```python
from build123d import *

# Parameters (mm, degrees)
BOSS_EXTRUDE1_DEPTH = 3
BOSS_EXTRUDE2_DEPTH = 15
BOSS_EXTRUDE3_DEPTH = 3
SKETCH5_R           = 2.25
CUT_EXTRUDE1_DEPTH  = 3
SKETCH6_R           = 2.6
CUT_EXTRUDE2_DEPTH  = 3
FILLET1_R           = 1


with BuildPart() as part:
    # Sketch2 → Boss-Extrude1 (new body)
    with BuildSketch(Plane(origin=(0, 0, 0), x_dir=(0, 0, -1), z_dir=(1, 0, 0))):
        Polygon((0, 0), (0, 40), (-5, 40), (-19, 5), (-19, 0), align=None)
    extrude(amount=BOSS_EXTRUDE1_DEPTH)

    # Sketch3 → Boss-Extrude2 (add)
    with BuildSketch(Plane(origin=(3, 0, 0), x_dir=(0, 0, -1), z_dir=(1, 0, 0))):
        Polygon((-19, 0), (-19, 3), (-3, 3), (-3, 40), (0, 40), (0, 0), align=None)
    extrude(amount=BOSS_EXTRUDE2_DEPTH)

    # Sketch4 → Boss-Extrude3 (add)
    with BuildSketch(Plane(origin=(18, 0, 0), x_dir=(0, 0, -1), z_dir=(1, 0, 0))):
        Polygon((-19, 0), (0, 0), (0, 40), (-5, 40), (-19, 5), align=None)
    extrude(amount=BOSS_EXTRUDE3_DEPTH)

    # Sketch5 → Cut-Extrude1 (cut)
    with BuildSketch(Plane(origin=(0, 0, 0), x_dir=(-1, 0, 0), z_dir=(0, 0, -1))):
        with Locations((-10.5, 30.5)):
            Circle(SKETCH5_R)
    extrude(amount=-CUT_EXTRUDE1_DEPTH, mode=Mode.SUBTRACT)

    # Sketch6 → Cut-Extrude2 (cut)
    with BuildSketch(Plane.XZ):
        with Locations(Location((10.5, 10, 0), (0, 0, 270))):
            Circle(SKETCH6_R)
    extrude(amount=-CUT_EXTRUDE2_DEPTH, mode=Mode.SUBTRACT)

    # Fillet1
    fillet1_edges = [part.edges().sort_by_distance(p)[0] for p in [
        (3, 22.5, 12),
        (3, 4, 19),
        (3, 40, 4),
        (3, 21.5, 3),
        (10.5, 40, 3),
        (3, 3, 11),
        (10.5, 3, 19),
        (18, 21.5, 3),
        (18, 3, 11),
        (18, 40, 4),
        (18, 22.5, 12),
        (18, 4, 19),
        (21, 20, 0),
        (21, 40, 2.5),
        (21, 22.5, 12),
        (21, 2.5, 19),
        (21, 0, 9.5),
        (0, 2.5, 19),
        (12.75, 30.5, 0),
        (0, 22.5, 12),
        (10.5, 0, 12.6),
        (0, 40, 2.5),
        (0, 20, 0),
        (0, 0, 9.5),
        (10.5, 0, 19),
        (10.5, 40, 0),
        (10.5, 0, 0),
    ]]
    fillet(fillet1_edges, radius=FILLET1_R)


solid = part.part
```
Source: CAD feature listing. Evaluate the final solid. Frame: model axes, mm. A direction names the side the tool comes from. Give positions to 0.01 mm unless a question says otherwise; leave off trailing zeros. Loops run counter-clockwise (first coordinate to the right, second up) from the corner with the lowest first, then second, coordinate; pieces in that order, holes last. Notation, with made-up numbers: (60, 29.25) -> (109, 29.25) arc R16 cw to (109, 33.25) -> close; hole circle Ø11 at (74, 57). An arc over 180 degrees is marked (long way). Use a Markdown table: item, result. Add a question column.
(1) Ray query, line 1 (X direction, y = 23, z = 6.75); line 2 (X direction, y = 2.45, z = 10); line 3 (Y direction, x = 5.5, z = 6.75). Return the intervals inside material, ascending.
(2) First-contact query: pin 1 Ø4 at (x, z) = (8.5, 13) entering from +Y; pin 2 Ø8 at (x, y) = (9.5, 33) entering from +Z; pin 3 Ø6 at (x, z) = (18.5, 9) entering from -Y; pin 4 Ø6 at (x, z) = (10.5, 10) entering from -Y. Flat tips, straight axial feed; report the tip coordinate or a pass-through.
(3) Section query B-B (x = 5). Output: boundary loops of the cut face in (y, z), then the cut area to 3 significant figures.
(4) Section query A-A (x = 10.5). Output: boundary loops of the cut face in (y, z), then the cut area to 3 significant figures.
(5) Access query for faces 1 (the face through (0.301, 2.972, 18.715)), 2 (the face through (2.699, 4.493, 18.715)). Directions: +Z, -Z, +X, -X, +Y, -Y. A direction counts if a zero-diameter tool reaches every point of the face in a straight line with its end or side. Return the directions, or none.
(6) Pull-direction query (X, two-part tool) for faces 3 (the face through (1.493, 22.745, 11.902)), 4 (the face through (21, 16, 8)), 5 (the face through (2.7, 22.15, 11.83)), 6 (the face through (8.193, 1.986, 8.8)); classes: +X half, -X half, draft (parallel to the pull), parting line (faces both ways), or undercut.
Checked values:
| question | item | result |
|---|---|---|
| 1 | line 1 | 0 to 3, 18 to 21 |
| 1 | line 2 | 0 to 7.9, 13.1 to 21 |
| 1 | line 3 | 0 to 3 |
| 2 | pin 1 | y = 3 |
| 2 | pin 2 | z = 3 |
| 2 | pin 3 | y = 0 |
| 2 | pin 4 | y = 0.2 |
| 3 | outline | (0, 1) arc R1 ccw to (1, 0) -> (39, 0) arc R1 ccw to (40, 1) -> (40, 2) arc R1 ccw to (39, 3) -> (3, 3) -> (3, 18) arc R1 ccw to (2, 19) -> (1, 19) arc R1 ccw to (0, 18) -> close |
| 3 | area | 167 mm^2 |
| 4 | outline | (0, 1) arc R1 ccw to (1, 0) -> (27.25, 0) arc R1 ccw to (28.25, 1) -> (28.25, 3) -> (3, 3) -> (3, 7.4) -> (1, 7.4) arc R1 ccw to (0, 6.4) -> close; (0, 13.6) arc R1 ccw to (1, 12.6) -> (3, 12.6) -> (3, 18) arc R1 ccw to (2, 19) -> (1, 19) arc R1 ccw to (0, 18) -> close; (32.75, 1) arc R1 ccw to (33.75, 0) -> (39, 0) arc R1 ccw to (40, 1) -> (40, 2) arc R1 ccw to (39, 3) -> (32.75, 3) -> close |
| 4 | area | 137 mm^2 |
| 5 | face 1 | +Z, -X, +Y, -Y |
| 5 | face 2 | +Z, +Y |
| 6 | face 3 | draft |
| 6 | face 4 | +X half |
| 6 | face 5 | undercut |
| 6 | face 6 | undercut |
